Geometry check sheet. Reference: the model listing, model coordinates, mm. A direction names the side the tool comes from. Round coordinates to 2 decimals unless told otherwise and drop trailing zeros. Write each loop counter-clockwise with the first axis right and the second up, starting at its lowest first coordinate (ties: lowest second). Pieces come first, ordered by that corner, then holes.
from build123d import *

# Parameters (mm, degrees)
EXTRUSION1_DEPTH = 80
ESQUISSE2_R      = 1.5
EXTRUSION2_DEPTH = 80


with BuildPart() as part:
    # Esquisse1 → Extrusion1 (new body)
    with BuildSketch(Plane.XY):
        Polygon((-29.286808535, 12.129808714), (-29.286808535, 10.629808714), (-9.286808535, 10.629808714), (-9.286808535, 30.629808714), (-10.786808535, 30.629808714), (-10.786808535, 12.129808714), align=None)
    extrude(amount=EXTRUSION1_DEPTH)

    # Esquisse2 → Extrusion2 (cut)
    with BuildSketch(Plane.XZ.offset(-10.629808714)):
        with Locations(Location((-14.286808535, 74, 0), (0, 0, 270))):
            Circle(ESQUISSE2_R)
        with Locations(Location((-24.286808535, 74, 0), (0, 0, 270))):
            Circle(ESQUISSE2_R)
        with Locations(Location((-14.286808535, 16, 0), (0, 0, 270))):
            Circle(ESQUISSE2_R)
        with Locations(Location((-24.286808535, 10, 0), (0, 0, 270))):
            Circle(ESQUISSE2_R)
        with Locations(Location((-19.286808535, 40, 0), (0, 0, 270))):
            Circle(ESQUISSE2_R)
    extrude(amount=-EXTRUSION2_DEPTH, mode=Mode.SUBTRACT)


solid = part.part
1. Section check C-C (z = 74). Record the cut outline in (x, y), plus the area to 4 significant figures.
2. Scan lines: line 1 along X through (y, z) = (11.2, 74); line 2 along X through (y, z) = (11.55, 10); line 3 along X through (y, z) = (11.65, 16). Record each from-to range of solid material in increasing order.
3. Access from +Z, -Z, +X, -X, +Y, -Y to the whole of each face (thin tool, end or side, straight path). Record for faces 4 (the face through (-10.787, 22, 39)), 5 (the face through (-29.287, 11, 39)).
4. Section check B-B (x = -20). Record the cut outline in (y, z).
5. Release check for a two-part mould opening along Z. For faces 1 (the face through (-14.9, 11.8, 0)), 2 (the face through (-19.22, 11.37, 41.5)), 3 (the face through (-17, 10.63, 39)) record: +Z half, -Z half, draft (parallel to the pull), parting line (faces both ways), or undercut.
6. Section check A-A (z = 16). Record the cut outline in (x, y).
7. Section check D-D (y = 18). Record the cut outline in (x, z), plus the area to 3 significant figures.
8. Depth check by flat-ended pin: pin 1 Ø4 at (x, y) = (-18, 15.5) entering from +Z; pin 2 Ø4 at (x, z) = (-14.29, 16) entering from +Y; pin 3 Ø1 at (y, z) = (16, 60.5) entering from -X. Enter the tip coordinate at first touch or a pass-through.
Results below:
1. outline: (-29.29, 10.63) - (-25.79, 10.63) - (-25.79, 12.13) - (-29.29, 12.13) - close; (-22.79, 10.63) - (-15.79, 10.63) - (-15.79, 12.13) - (-22.79, 12.13) - close; (-12.79, 10.63) - (-9.29, 10.63) - (-9.29, 30.63) - (-10.79, 30.63) - (-10.79, 12.13) - (-12.79, 12.13) - close
1. area: 48.75 mm2
2. line 1: x = -29.29 to -25.79, -22.79 to -15.79, -12.79 to -9.29
2. line 2: x = -29.29 to -25.79, -22.79 to -9.29
2. line 3: x = -29.29 to -15.79, -12.79 to -9.29
3. face 4: +Z, -Z, -X, +Y
3. face 5: +Z, -Z, -X, +Y, -Y
4. outline: (10.63, 0) - (12.13, 0) - (12.13, 38.68) - (10.63, 38.68) - close; (10.63, 41.32) - (12.13, 41.32) - (12.13, 80) - (10.63, 80) - close
5. face 1: -Z half
5. face 2: undercut
5. face 3: draft
6. outline: (-29.29, 10.63) - (-15.79, 10.63) - (-15.79, 12.13) - (-29.29, 12.13) - close; (-12.79, 10.63) - (-9.29, 10.63) - (-9.29, 30.63) - (-10.79, 30.63) - (-10.79, 12.13) - (-12.79, 12.13) - close
7. outline: (-10.79, 0) - (-9.29, 0) - (-9.29, 80) - (-10.79, 80) - close
7. area: 120 mm2
8. pin 1: passes through
8. pin 2: stops at y = 12.13
8. pin 3: stops at x = -10.79
